```python
from build123d import *

# Parameters (mm, degrees)
SKETCH1_W           = 120
SKETCH1_H           = 60
BOSS_EXTRUDE1_DEPTH = 120
SKETCH2_W           = 10
SKETCH2_H           = 30
CUT_EXTRUDE1_DEPTH  = 120
SKETCH3_W           = 10
SKETCH3_H           = 20
CUT_EXTRUDE2_DEPTH  = 120
CUT_EXTRUDE3_DEPTH  = 120
SKETCH6_R           = 20
CUT_EXTRUDE4_DEPTH  = 120
CUT_EXTRUDE5_DEPTH  = 20
CUT_EXTRUDE8_DEPTH  = 20
SKETCH9_W           = 15
SKETCH9_H           = 10
CUT_EXTRUDE10_DEPTH = 20
SKETCH10_W          = 29.72135955
SKETCH10_H          = 10
CUT_EXTRUDE11_DEPTH = 20
CUT_EXTRUDE12_DEPTH = 20
SKETCH12_W          = 40
SKETCH12_H          = 20
CUT_EXTRUDE15_DEPTH = 20
SKETCH14_W          = 20
SKETCH14_H          = 40
BOSS_EXTRUDE6_DEPTH = 20


with BuildPart() as part:
    # Sketch1 → Boss-Extrude1 (new body)
    with BuildSketch(Plane.XY):
        with Locations((60, 30)):
            Rectangle(SKETCH1_W, SKETCH1_H)
    extrude(amount=BOSS_EXTRUDE1_DEPTH)

    # Sketch2 → Cut-Extrude1 (cut)
    with BuildSketch(Plane.XY.offset(120)):
        with Locations((5, 45)):
            Rectangle(SKETCH2_W, SKETCH2_H)
    extrude(amount=-CUT_EXTRUDE1_DEPTH, mode=Mode.SUBTRACT)

    # Sketch3 → Cut-Extrude2 (cut)
    with BuildSketch(Plane.XY.offset(120)):
        with Locations((15, 50)):
            Rectangle(SKETCH3_W, SKETCH3_H)
    extrude(amount=-CUT_EXTRUDE2_DEPTH, mode=Mode.SUBTRACT)

    # Sketch5 → Cut-Extrude3 (cut)
    with BuildSketch(Plane.XZ):
        with BuildLine():
            Line((60, 120), (0, 120))
            Line((0, 120), (0, 60))
            ThreePointArc((0, 60), (17.573593129, 102.426406871), (60, 120))
        make_face()
        with BuildLine():
            Line((120, 120), (60, 120))
            ThreePointArc((60, 120), (102.426406871, 102.426406871), (120, 60))
            Line((120, 60), (120, 120))
        make_face()
        with BuildLine():
            ThreePointArc((120, 60), (102.426406871, 17.573593129), (60, 0))
            Line((60, 0), (120, 0))
            Line((120, 0), (120, 60))
        make_face()
        with BuildLine():
            ThreePointArc((60, 0), (17.573593129, 17.573593129), (0, 60))
            Line((0, 60), (0, 0))
            Line((0, 0), (60, 0))
        make_face()
    extrude(amount=-CUT_EXTRUDE3_DEPTH, mode=Mode.SUBTRACT)

    # Sketch6 → Cut-Extrude4 (cut)
    with BuildSketch(Plane(origin=(0, 0, 0), x_dir=(-1, 0, 0), z_dir=(0, -1, 0))):
        with Locations((-60, -60)):
            Circle(SKETCH6_R)
    extrude(amount=-CUT_EXTRUDE4_DEPTH, mode=Mode.SUBTRACT)

    # Sketch7 → Cut-Extrude5 (cut)
    with BuildSketch(Plane(origin=(0, 60, 0), x_dir=(1, 0, 0), z_dir=(0, 1, 0))):
        with BuildLine():
            Line((40, -60), (40, -116.568542495))
            ThreePointArc((40, -116.568542495), (60, -120), (80, -116.568542495))
            Line((80, -116.568542495), (80, -60))
            ThreePointArc((80, -60), (60, -80), (40, -60))
        make_face()
    extrude(amount=-CUT_EXTRUDE5_DEPTH, mode=Mode.SUBTRACT)

    # Sketch8 → Cut-Extrude8 (cut)
    with BuildSketch(Plane(origin=(0, 60, 0), x_dir=(1, 0, 0), z_dir=(0, 1, 0))):
        with BuildLine():
            ThreePointArc((100, -60), (88.284271247, -31.715728753), (60, -20))
            Line((60, -20), (20, -20))
            Line((20, -20), (20, -104.72135955))
            ThreePointArc((20, -104.72135955), (29.420776074, -111.622776602), (40, -116.568542495))
            Line((40, -116.568542495), (40, -60))
            ThreePointArc((40, -60), (60, -40), (80, -60))
            Line((80, -60), (80, -116.568542495))
            ThreePointArc((80, -116.568542495), (90.579223926, -111.622776602), (100, -104.72135955))
            Line((100, -104.72135955), (100, -60))
        make_face()
    extrude(amount=-CUT_EXTRUDE8_DEPTH, mode=Mode.SUBTRACT)

    # Sketch9 → Cut-Extrude10 (cut)
    with BuildSketch(Plane.ZY.offset(-100)):
        with Locations((97.22135955, 55)):
            Rectangle(SKETCH9_W, SKETCH9_H)
    extrude(amount=-CUT_EXTRUDE10_DEPTH, mode=Mode.SUBTRACT)

    # Sketch10 → Cut-Extrude11 (cut)
    with BuildSketch(Plane.ZY.offset(-100)):
        with Locations((74.860679775, 55)):
            Rectangle(SKETCH10_W, SKETCH10_H)
    extrude(amount=-CUT_EXTRUDE11_DEPTH, mode=Mode.SUBTRACT)

    # Sketch11 → Cut-Extrude12 (cut)
    with BuildSketch(Plane(origin=(0, 40, 0), x_dir=(1, 0, 0), z_dir=(0, 1, 0))):
        with BuildLine():
            Line((40, -60), (40, -116.568542495))
            ThreePointArc((40, -116.568542495), (60, -120), (80, -116.568542495))
            Line((80, -116.568542495), (80, -60))
            ThreePointArc((80, -60), (60, -80), (40, -60))
        make_face()
    extrude(amount=-CUT_EXTRUDE12_DEPTH, mode=Mode.SUBTRACT)

    # Sketch12 → Cut-Extrude15 (cut)
    with BuildSketch(Plane(origin=(40, 0, 0), x_dir=(0, 0, -1), z_dir=(1, 0, 0))):
        with Locations((-60, 30)):
            Rectangle(SKETCH12_W, SKETCH12_H)
    extrude(amount=-CUT_EXTRUDE15_DEPTH, mode=Mode.SUBTRACT)

    # Sketch14 → Boss-Extrude6 (add)
    with BuildSketch(Plane(origin=(0, 40, 0), x_dir=(1, 0, 0), z_dir=(0, 1, 0))):
        with Locations((30, -60)):
            Rectangle(SKETCH14_W, SKETCH14_H)
    extrude(amount=-BOSS_EXTRUDE6_DEPTH)


solid = part.part
```
Check sheet for the modelled part. Datum: model origin and axes. Units: mm. A direction names the side the tool comes from. Give positions to 0.01 mm unless a question says otherwise; leave off trailing zeros. Loops run counter-clockwise (first coordinate to the right, second up) from the corner with the lowest first, then second, coordinate; pieces in that order, holes last. Notation, with made-up numbers: (15, 88.5) - (46, 88.5) arc R17 ccw to (46, 108.5) - close; hole circle Ø2 at (-35.5, 9). An arc over 180 degrees is marked (long way). One line per question, with ' | ' between items. Start each with the question number.
1. Cross-section at C-C, the plane z = 102.5. Enter the section's corners in (x, y).
2. Cross-section at B-B, the plane x = 67. Enter the section's corners in (y, z) (3 decimals), plus the area to 3 significant figures.
3. Draft check along X on faces 1 (the flat face through (60, 20, 96)), 2 (the flat face through (110, 55, 60)), 3 (the flat face through (10, 35, 60)), 4 (the flat face through (40, 30, 89)). Enter one of: released by +X, released by -X, zero draft, split by the parting line, or undercut.
4. Cross-section at D-D, the plane y = 7. Enter the section's corners in (x, z).
5. Cross-section at A-A, the plane y = 23.5. Enter the section's corners in (x, z), plus the area to 3 significant figures.
6. Material ranges on line 1 along X through (y, z) = (9.5, 60); line 2 along X through (y, z) = (38.5, 55), recorded low to high. Write a range as [from, to].
7. Gauge pin test, flat ends, axial feed: pin 1 Ø3 at (y, z) = (10, 73.5) entering from -X; pin 2 Ø2 at (y, z) = (54, 55) entering from -X; pin 3 Ø1.5 at (x, y) = (47, 27) entering from -Z. Record the tip position at first contact, or that the pin passes through.
8. Set-up check for faces 5 (the flat face through (20, 50, 18)), 6 (the flat face through (80, 30, 89)), 7 (the cylindrical face through (88.594, 50.14, 32.028)), 8 (the flat face through (108, 50, 77)), 9 (the flat face through (77, 60, 21)): record each of +Z, -Z, +X, -X, +Y, -Y from which the full face is reachable in a straight line by a thin tool's end or side.
Check result:
1) outline: (17.65, 0) - (102.35, 0) - (102.35, 50) - (100, 50) - (100, 40) - (80, 40) - (80, 20) - (40, 20) - (40, 40) - (17.65, 40) - close
2) outline: (0, 0.41) - (60, 0.41) - (60, 20.617) - (40, 20.617) - (40, 41.265) - (0, 41.265) - close; (0, 78.735) - (20, 78.735) - (20, 119.59) - (0, 119.59) - close | area: 2,860 mm2
3) face 1: undercut | face 2: zero draft | face 3: released by -X | face 4: undercut
4) outline: circle Ø120 at (60, 60); hole circle Ø40 at (60, 60)
5) outline: (40, 60) - (40, 116.57) arc R60 ccw (long way) to (80, 116.57) - (80, 60) arc R20 cw to start | area: 8,330 mm2
6) line 1: x = [0, 40], [80, 120] | line 2: x = [10, 40.64], [79.36, 119.79]
7) pin 1: stops at x = 1.21 | pin 2: stops at x = 99.55 | pin 3: stops at z = 1.26
8) face 5: +Z, -Z, -X, +Y | face 6: +Z, +Y | face 7: +Z, -X, +Y | face 8: +Z, +X, -X, +Y | face 9: +Z, -Z, +X, -X, +Y
